Part model, mm, in its own coordinate system. A direction names the side the tool comes from. Round coordinates to 2 decimals unless told otherwise and drop trailing zeros. Write each loop counter-clockwise with the first axis right and the second up, starting at its lowest first coordinate (ties: lowest second). Pieces come first, ordered by that corner, then holes. Notation, with made-up numbers: (37, 81.5) -> (62, 81.5) arc R8 cw to (62, 90.5) -> close; hole circle Ø6 at (75.25, 35). An arc over 180 degrees is marked (long way). Use CSV: the item, a comma, the result in double quotes. Start each with the question number.
Autodesk Inventor part; units mm, degrees
ref_plane "YZ Plane" through (0, 0, 0) normal (1, 0, 0) x (0, 1, 0)
ref_plane "XZ Plane" through (0, 0, 0) normal (0, 1, 0) x (-1, 0, 0)
ref_plane "XY Plane" through (0, 0, 0) normal (0, 0, 1) x (1, 0, 0)
sketch "Esquisse1" plane through (0, 0, 0) normal (0, 0, 1) x (1, 0, 0)
  circle A0 centre (0, 0) radius 30
  circle A1 centre (0, 0) radius 27
  dimension "d0" = 60
  dimension "d1" = 54
extrude "Extrusion1" add sketch "Esquisse1" along normal blind 32
sketch "Esquisse2" plane through (0, 0, 0) normal (0, 1, 0) x (-1, 0, 0)
  circle A0 centre (0, 16.4966) radius 15.5
  circle A1 centre (0, 16.4966) radius 12
  point P0 (0, 0)
  dimension "d18" = 24
  dimension "d19" = 31
extrude "Extrusion2" cut sketch "Esquisse2" along normal blind 111.75 contours A1
thread "Filetage1"
sketch "Esquisse3" plane through (0, 0, 0) normal (1, 0, 0) x (0, 1, 0)
  line L0 (11.9576, 21.526) -> (-8.0424, 21.526)
  line L1 (-8.0424, 21.526) -> (-8.0424, 11.526)
  line L2 (-8.0424, 11.526) -> (11.9576, 11.526)
  line L3 (11.9576, 11.526) -> (11.9576, 21.526)
  line L4 (0, 0) -> (0, 32)
  line L5 (30, 0) -> (-30, 0)
  dimension "d10" = 10
  dimension "d12" = 32
  dimension "d17" = 20
extrude "Extrusion3" cut sketch "Esquisse3" along normal blind 30
properties part number "Cadran base"
1. Pull direction Z, two halves, no side cores. Call faces 1 (the flat face through (-25, 11, 32)), 2 (the flat face through (-25, 11, 0)), 3 (the flat face through (27, -8.042, 17)), 4 (the flat face through (26, 11.958, 16)): released by +Z, released by -Z, zero draft, split by the parting line, or undercut.
2. Flat gauge pins, fed straight in: pin 1 (5 mm diameter, centred on x = 14, z = 24.5, fed in from -Y); pin 2 (12 mm diameter, centred on x = 16, z = 17, fed in from -Y); pin 3 (5 mm diameter, centred on y = 12.5, z = 17.5, fed in from +X). Where does each tip first touch, or does it go through?
3. Drill centre lines: line 1 along Z through (x, y) = (0, 28); line 2 along X through (y, z) = (-21, 2); line 3 along X through (y, z) = (-8.5, 19). Where is each one in solid material? Low to high. Write a range as [from, to].
4. Which spindle directions (+Z, -Z, +X, -X, +Y, -Y) get a long thin tool onto all of the face, cutting with end or side? Do faces 5 (the cylindrical face through (-3.905, -29.745, 15.776)), 6 (the cylindrical face through (-6.451, 27.053, 6.378)), 7 (the flat face through (28, 2, 11.526)). Say none if no direction does.
5. Band-saw the part on A-A (x = 0). List the corners of the cut face in (y, z), then the cut area to 3 significant figures.
6. Band-saw the part on C-C (z = 13.5). List the corners of the cut face in (x, y), then the cut area to 3 significant figures.
7. Band-saw the part on D-D (x = 22). List the corners of the cut face in (y, z), then the cut area to 3 significant figures.
8. Band-saw the part on B-B (y = 0). List the corners of the cut face in (x, z), then the cut area to 3 significant figures.
Answers below:
1,face 1,"released by +Z"
1,face 2,"released by -Z"
1,face 3,"undercut"
1,face 4,"undercut"
2,pin 1,"stops at y = -27.71"
2,pin 2,"stops at y = -28.28"
2,pin 3,"stops at x = 27.51"
3,line 1,"z = [0, 4.5], [28.5, 32]"
3,line 2,"x = [-21.42, -16.97], [16.97, 21.42]"
3,line 3,"x = [-28.77, -25.63], [25.63, 28.77]"
4,face 5,"+Z, -Z"
4,face 6,"+Y"
4,face 7,"+X"
5,outline,"(-30, 0) -> (-27, 0) -> (-27, 32) -> (-30, 32) -> close; (27, 0) -> (30, 0) -> (30, 4.5) -> (27, 4.5) -> close; (27, 28.5) -> (30, 28.5) -> (30, 32) -> (27, 32) -> close"
5,area,"120 mm^2"
6,outline,"(-11.62, 24.37) -> (-11.62, 27.66) arc R30 ccw (long way) to (28.9, -8.04) -> (25.77, -8.04) arc R27 cw (long way) to start; (11.62, 24.37) arc R27 cw to (24.21, 11.96) -> (27.51, 11.96) arc R30 ccw to (11.62, 27.66) -> close"
6,area,"404 mm^2"
7,outline,"(-20.4, 0) -> (-15.65, 0) -> (-15.65, 32) -> (-20.4, 32) -> close; (15.65, 0) -> (20.4, 0) -> (20.4, 32) -> (15.65, 32) -> close"
7,area,"304 mm^2"
8,outline,"(-30, 0) -> (-27, 0) -> (-27, 32) -> (-30, 32) -> close; (27, 0) -> (30, 0) -> (30, 11.53) -> (27, 11.53) -> close; (27, 21.53) -> (30, 21.53) -> (30, 32) -> (27, 32) -> close"
8,area,"162 mm^2"
